Autodesk Inventor part; units mm, degrees
ref_plane "YZ Plane" through (0, 0, 0) normal (1, 0, 0) x (0, 1, 0)
ref_plane "XZ Plane" through (0, 0, 0) normal (0, 1, 0) x (-1, 0, 0)
ref_plane "XY Plane" through (0, 0, 0) normal (0, 0, 1) x (1, 0, 0)
sketch "Szkic1" plane through (0, 0, 0) normal (0, 1, 0) x (-1, 0, 0)
  circle A0 centre (0, 0) radius 10
  dimension "d0" = 20
extrude "Wyciągnięcie proste1" add sketch "Szkic1" along normal blind 400
shell "Skorupa1" thickness 2 removed faces 2 at (1.182, 0, 3.1167) at (1.182, 400, 3.1167)
sketch "Szkic2" plane through (0, 0, 0) normal (0, 0, 1) x (1, 0, 0)
  line L0 (-10, 0) -> (10, 0) construction
  line L1 (-10, 0) -> (10, 0)
  line L2 (22.37, 2.832) -> (-10, 0)
  line L3 (10, 0) -> (22.37, 2.832)
  line L4 (10, 400) -> (-10, 400) construction
  line L5 (10, 0) -> (10, 400) construction
  line L6 (-10, 400) -> (10, 400)
  line L7 (10, 400) -> (10, 398.2502)
  line L8 (10, 398.2502) -> (-10, 400)
  point P0 (0, 0)
  dimension "d4" = 5
  dimension "d7" = 5
extrude "Wyciągnięcie proste3" cut sketch "Szkic2" along normal mid plane 32
equation "\"PromieńGięcia\" = Grubość"
equation "\"SzerokośćGięciaPodcięcia\" = Grubość"
equation "\"GłębokośćGięciaPodcięcia\" = 0.5 * Grubość"
equation "\"RozmiarPodcięciaNarożnika\" = 4 * Grubość"
equation "\"MinimalnaPozostałość\" = 2 * Grubość"
equation "\"PromieńPrzejścia\" = PromieńGięcia"
equation "\"Rozmiar_promienia_Jacobiego\" = Grubość"
equation "\"Wielk_odstępu\" = Grubość"
properties part number "Rura_poprzeczna_ergosiedziska" material "Aluminium AW-7020"
Model file for the job. Use its own axes, mm. Coordinates: 2 decimals unless noted, no trailing zeros. Order: outer loops, then holes, each group sorted by start corner. A loop starts at its lowest first (then second) coordinate and runs counter-clockwise, first axis right, second up. Notation, with made-up numbers: M -34,-24.75 L -20,-24.75 A11 ccw -20,-13.75 Z; hole C 48.25,63.5 d2. An arc over 180 degrees is marked long. Answer as CSV lines item,"result".
(1) Flat gauge pins, fed straight in: pin 1 (8 mm diameter, centred on x = -2, y = 359.5, fed in from +Z); pin 2 (12 mm diameter, centred on x = -7.5, y = 51.5, fed in from -Z); pin 3 (12 mm diameter, centred on y = 82, z = -7.5, fed in from -X); pin 4 (8 mm diameter, centred on y = 205.5, z = 6, fed in from +X). Where does each tip first touch, or does it go through?
Geometry says:
pin 1,"stops at z = 10"
pin 2,"stops at z = -9.89"
pin 3,"stops at x = -9.89"
pin 4,"stops at x = 9.8"
(2) Band-saw the part on C-C, the plane y = 89.5. List the corners of the cut face in (x, z), then the cut area to 3 significant figures.
Geometry says:
outline,"C 0,0 d20; hole C 0,0 d16"
area,"113 mm2"
(3) Band-saw the part on B-B, the plane z = -3.5. List the corners of the cut face in (x, y), then the cut area to 3 significant figures.
Geometry says:
outline,"M -9.37,0.06 L -7.19,0.25 L -7.19,399.75 L -9.37,399.94 Z; M 7.19,1.5 L 9.37,1.69 L 9.37,398.31 L 7.19,398.5 Z"
area,"1,730 mm2"
(4) Pull direction X, two halves, no side cores. Call faces 1 (the cylindrical face through (1.73, 197.2, 7.81)), 2 (the flat face through (0.05, 399.12, -8.19)), 3 (the cylindrical face through (2.17, 197.2, 9.76)): +X half, -X half, draft (parallel to the pull), parting line (faces both ways), or undercut.
Geometry says:
face 1,"undercut"
face 2,"+X half"
face 3,"parting line"
(5) Band-saw the part on A-A, the plane x = 4.25. List the corners of the cut face in (y, z).
Geometry says:
outline,"M 1.25,-9.05 L 398.75,-9.05 L 398.75,-6.78 L 1.25,-6.78 Z; M 1.25,6.78 L 398.75,6.78 L 398.75,9.05 L 1.25,9.05 Z"
(6) Wall check: line 1 along Z through (x, y) = (0.25, 379); line 2 along Z through (x, y) = (3.75, 48.5). Give the ranges that are in metal, low to high.
Geometry says:
line 1,"z = -10 to -8, 8 to 10"
line 2,"z = -9.27 to -7.07, 7.07 to 9.27"
